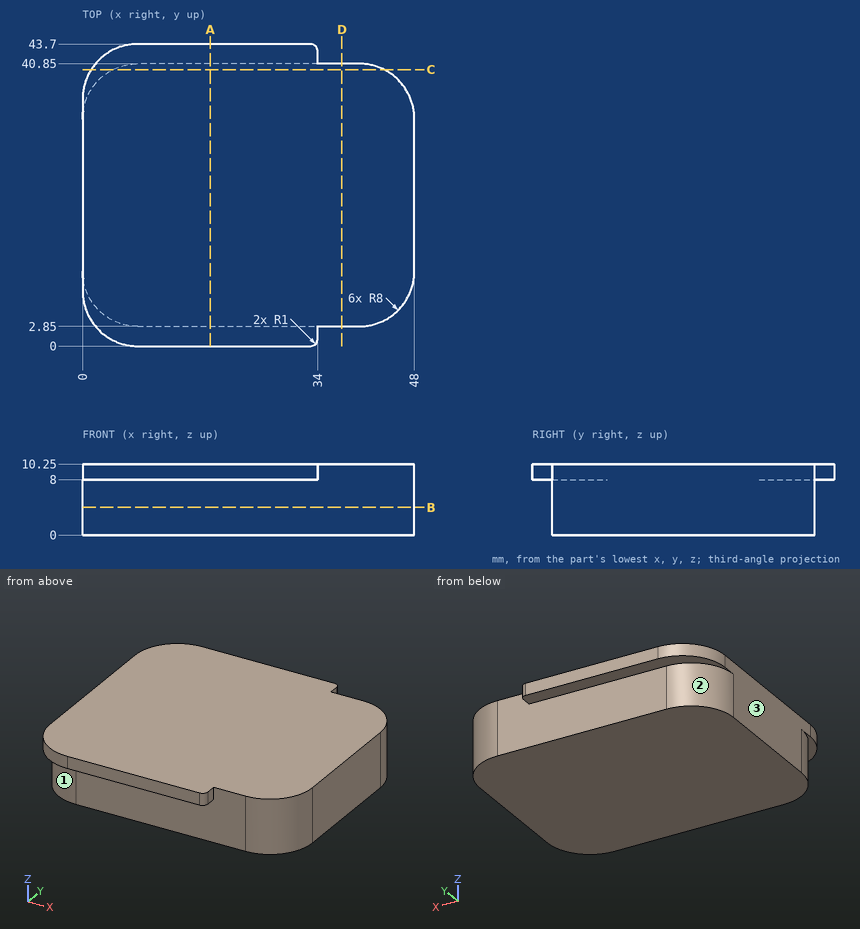
For this review, use the dimensioned drawing (mm, ordinates from the lowest corner) and the shaded views. Round coordinates to 2 decimals unless told otherwise and drop trailing zeros. Write each loop counter-clockwise with the first axis right and the second up, starting at its lowest first coordinate (ties: lowest second). Pieces come first, ordered by that corner, then holes. Notation, with made-up numbers: (34.25, -10) - (56.25, -10) arc R33 cw to (56.25, 23) - close; hole circle Ø11 at (60.5, -13). An arc over 180 degrees is marked (long way). One line per item, written item: value. Start each with the question number.
1. Consider section C-C on y = 40. Write out the cut boundary in (x, z).
2. Consider section D-D on x = 37.5. Write out the cut boundary in (y, z).
3. Clearance check with flat-ended pins moving along their axes: P1, Ø3, axis at y = 36.5, z = 4, coming from the +X side; P2, Ø3, axis at x = 9, z = 2.5, coming from the +Y side; P3, Ø6, axis at y = 38.5, z = 3.5, coming from the +X side. State where each tip first meets the part, or that it passes through.
4. Consider section B-B on z = 4. Write out the cut boundary in (x, y).
5. To check wall thickness, follow L1, parallel to Y at x = 25.5, z = 4; L2, parallel to Z at x = 4, y = 42; L3, parallel to X at y = 9, z = 1.75. State the ranges of each line that lie inside material, in increasing order. Write a range as from..to.
6. The part is to be moulded in two halves that separate along Y. For the marked faces 1, 2 and 3, say which applies: released by +Y, released by -Y, zero draft, split by the parting line, or undercut.
7. Consider section A-A on x = 18.5. Write out the cut boundary in (y, z).
Checks:
1. outline: (1.25, 8) - (4.41, 8) - (4.41, 0) - (43.59, 0) - (43.59, 10.25) - (1.25, 10.25) - close
2. outline: (2.85, 0) - (40.85, 0) - (40.85, 10.25) - (2.85, 10.25) - close
3. P1: stops at x = 47.71
3. P2: stops at y = 40.85
3. P3: stops at x = 47.55
4. outline: (0, 10.85) arc R8 ccw to (8, 2.85) - (40, 2.85) arc R8 ccw to (48, 10.85) - (48, 32.85) arc R8 ccw to (40, 40.85) - (8, 40.85) arc R8 ccw to (0, 32.85) - close
5. L1: y = 2.85..40.85
5. L2: z = 8..10.25
5. L3: x = 0.22..47.78
6. face 1: released by -Y
6. face 2: released by +Y
6. face 3: zero draft
7. outline: (0, 8) - (2.85, 8) - (2.85, 0) - (40.85, 0) - (40.85, 8) - (43.7, 8) - (43.7, 10.25) - (0, 10.25) - close
